Verification items for this drawing (mm, ordinates from the low corner). Round coordinates to 2 decimals unless told otherwise and drop trailing zeros. Loops run counter-clockwise (first coordinate to the right, second up) from the corner with the lowest first, then second, coordinate; pieces in that order, holes last. Notation, with made-up numbers: (49.5, 72) -> (56.5, 72) arc R11 cw to (56.5, 92) -> close; hole circle Ø6 at (38.5, -38). An arc over 180 degrees is marked (long way). Use a Markdown table: item, result. Add a question column.
Q1. Sectioned sample at C-C, the plane z = 0.65. Enter the section's corners in (x, y), then the cut area to 3 significant figures.
Q2. Gauge pin test, flat end, axial feed: P1, Ø2, axis at x = 13, y = 19.5, coming from the -Z side. Record the tip position at first contact, or that the pin passes through.
Q3. Sectioned sample at A-A, the plane y = 20.5. Enter the section's corners in (x, z), then the cut area to 3 significant figures.
Q4. Sectioned sample at B-B, the plane x = 22. Enter the section's corners in (y, z).
Q5. Material ranges on L1, parallel to X at y = 21, z = 0.55; L2, parallel to Y at x = 20.5, z = 0.45; L3, parallel to X at y = 33, z = 0.25, recorded low to high.
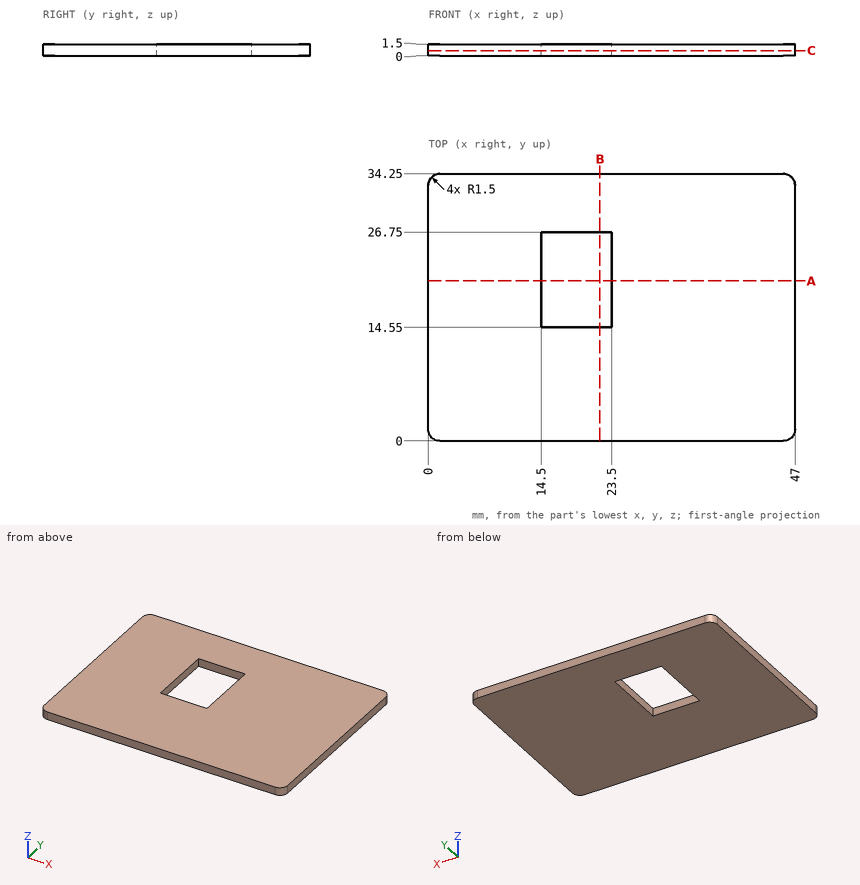
Values:
| question | item | result |
|---|---|---|
| 1 | outline | (0, 1.5) arc R1.5 ccw to (1.5, 0) -> (45.5, 0) arc R1.5 ccw to (47, 1.5) -> (47, 32.75) arc R1.5 ccw to (45.5, 34.25) -> (1.5, 34.25) arc R1.5 ccw to (0, 32.75) -> close; hole (14.5, 14.55) -> (23.5, 14.55) -> (23.5, 26.75) -> (14.5, 26.75) -> close |
| 1 | area | 1,500 mm^2 |
| 2 | P1 | z = 0 |
| 3 | outline | (0, 0) -> (14.5, 0) -> (14.5, 1.5) -> (0, 1.5) -> close; (23.5, 0) -> (47, 0) -> (47, 1.5) -> (23.5, 1.5) -> close |
| 3 | area | 57.0 mm^2 |
| 4 | outline | (0, 0) -> (14.55, 0) -> (14.55, 1.5) -> (0, 1.5) -> close; (26.75, 0) -> (34.25, 0) -> (34.25, 1.5) -> (26.75, 1.5) -> close |
| 5 | L1 | 0 to 14.5, 23.5 to 47 |
| 5 | L2 | 0 to 14.55, 26.75 to 34.25 |
| 5 | L3 | 0.02 to 46.98 |
